Verification items for the finished model (mm, model axes). Face numbers are marked on the shaded views. Give positions to 0.01 mm unless a question says otherwise; leave off trailing zeros. Write each loop counter-clockwise with the first axis right and the second up, starting at its lowest first coordinate (ties: lowest second). Pieces come first, ordered by that corner, then holes. Notation, with made-up numbers: (-34, 14.25) - (19, 14.25) arc R32 cw to (19, 53.25) - close; hole circle Ø9 at (4, 10.5). An arc over 180 degrees is marked (long way). Put each result on its own line as item: value.
from build123d import *


with BuildPart() as part:
    # Esquisse1 → Base-Révolution (revolve)
    with BuildSketch(Plane.XY, mode=Mode.PRIVATE) as base_r_volution_sk:
        with BuildLine():
            Line((1, 12.5), (24, 12.5))
            ThreePointArc((24, 12.5), (24.707106781, 12.792893219), (25, 13.5))
            Line((25, 13.5), (25, 22.5))
            Line((25, 22.5), (22.321383042, 22.499995211))
            ThreePointArc((22.321383042, 22.499995211), (17.738807347, 19.499995211), (13.156231652, 22.499995211))
            Line((13.156231652, 22.499995211), (11.22402651, 22.499995211))
            Line((11.22402651, 22.499995211), (11.232186751, 21.25))
            Line((11.232186751, 21.25), (8.732186751, 21.233679457))
            Line((8.732186751, 21.233679457), (8.732186751, 20))
            Line((8.732186751, 20), (1.732186751, 20))
            Line((1.732186751, 20), (1.732186751, 21.233679457))
            Line((1.732186751, 21.233679457), (0, 21.233679457))
            Line((0, 21.233679457), (0, 20))
            Line((0, 20), (0, 13.5))
            ThreePointArc((0, 13.5), (0.292893219, 12.792893219), (1, 12.5))
        make_face()
    revolve(base_r_volution_sk.sketch.rotate(Axis((0, 0, 0), (1, 0, 0)), 90), axis=Axis((0, 0, 0), (1, 0, 0)))


solid = part.part
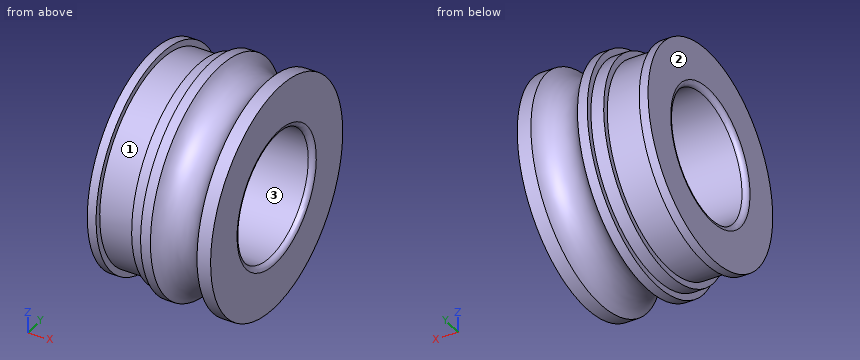
Q1. Section check B-B, the plane x = 12.5. Record the cut outline in (y, z), plus the area to 3 significant figures.
Answers follow:
outline: circle Ø45 at (0, 0); hole circle Ø25 at (0, 0)
area: 1,100 mm2
Q2. Go/stop test with flat-tipped pins: pin 1 Ø8 at (x, y) = (17, -3.5) entering from +Z; pin 2 Ø2 at (x, y) = (22.5, 5.5) entering from +Z; pin 3 Ø1 at (x, z) = (5.5, -2) entering from +Y. Record where each tip stops, or that it passes through.
Answers follow:
pin 1: stops at z = 22.37
pin 2: stops at z = 22.05
pin 3: stops at y = 19.94
Q3. Section check A-A, the plane x = 7. Record the cut outline in (y, z), plus the area to 3 significant figures.
Answers follow:
outline: circle Ø40 at (0, 0); hole circle Ø25 at (0, 0)
area: 766 mm2
Q4. Scan lines: line 1 along X through (y, z) = (19.5, 6.5); line 2 along Y through (x, z) = (10.75, 0); line 3 along Y through (x, z) = (22.75, 0.5). Record each from-to range of solid material in increasing order.
Answers follow:
line 1: x = 0 to 1.73, 8.73 to 14.67, 20.81 to 25
line 2: y = -21.25 to -12.5, 12.5 to 21.25
line 3: y = -22.49 to -12.49, 12.49 to 22.49
Q5. Release check for a two-part mould opening along Z. For the marked faces 1, 2 and 3 record: released by +Z, released by -Z, zero draft, split by the parting line, or undercut.
Answers follow:
face 1: split by the parting line
face 2: zero draft
face 3: undercut
